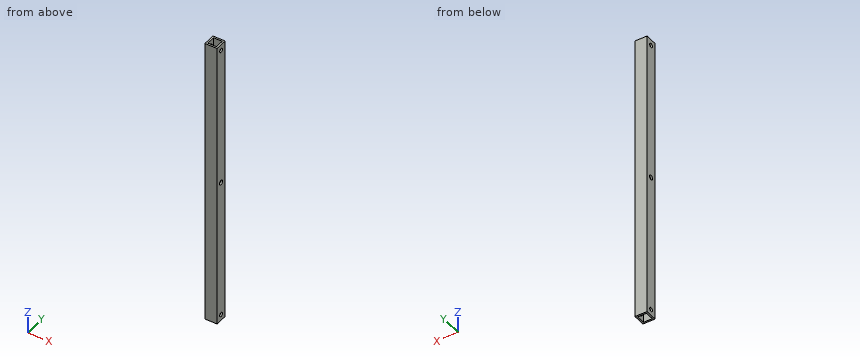
Autodesk Inventor part; units mm, degrees
ref_plane "YZ Plane" through (0, 0, 0) normal (1, 0, 0) x (0, 1, 0)
ref_plane "XZ Plane" through (0, 0, 0) normal (0, 1, 0) x (-1, 0, 0)
ref_plane "XY Plane" through (0, 0, 0) normal (0, 0, 1) x (1, 0, 0)
sketch "Sketch1" plane through (0, 0, 0) normal (0, 0, 1) x (1, 0, 0)
  line L0 (-6.35, -6.35) -> (6.35, -6.35)
  line L1 (6.35, -6.35) -> (6.35, 6.35)
  line L2 (6.35, 6.35) -> (-6.35, 6.35)
  line L3 (-6.35, 6.35) -> (-6.35, -6.35)
  line L4 (-6.35, -6.35) -> (6.35, 6.35) construction
  line L5 (6.35, -6.35) -> (-6.35, 6.35) construction
  line L6 (-4.572, -4.572) -> (4.572, -4.572)
  line L7 (4.572, -4.572) -> (4.572, 4.572)
  line L8 (4.572, 4.572) -> (-4.572, 4.572)
  line L9 (-4.572, 4.572) -> (-4.572, -4.572)
  line L10 (-4.572, -4.572) -> (4.572, 4.572) construction
  line L11 (4.572, -4.572) -> (-4.572, 4.572) construction
  point P0 (0, 0)
  dimension "d0" = 12.7
  dimension "d1" = 12.7
  dimension "d5" = 1.778
extrude "Extrusion1" add sketch "Sketch1" along normal blind 304.8
sketch "Sketch3" plane through (6.35, 6.35, 304.8) normal (1, 0, 0) x (0, 0, -1)
  point P0 (304.8, -6.35)
  point P1 (152.4, -6.35)
hole "Hole1" at (6.35, 0, 152.4) direction (-1, 0, 0) diameter 4.7625 depth 25.4 tip angle 118
sketch "Sketch4" plane through (-6.35, -6.35, 0) normal (-1, 0, 0) x (0, 0, 1)
  line L0 (0, 12.7) -> (0, 0)
  line L1 (304.8, 12.7) -> (304.8, 0)
  circle A0 centre (298.45, 6.35) radius 2.1336
  circle A1 centre (6.35, 6.35) radius 2.1336
  point P0 (0, 6.35)
  dimension "d13" = 4.2672
  dimension "d14" = 6.35
  dimension "d15" = 4.2672
  dimension "d16" = 6.35
extrude "Extrusion2" cut sketch "Sketch4" against normal blind 12.7
properties part number "5x5mm Box Aluminum" material "Aluminum 6061"
Part model, mm, in its own coordinate system. Give positions to 0.01 mm unless a question says otherwise; leave off trailing zeros. Loops run counter-clockwise (first coordinate to the right, second up) from the corner with the lowest first, then second, coordinate; pieces in that order, holes last. Notation, with made-up numbers: (5, 26) -> (18, 26) arc R25 ccw to (18, 55) -> close; hole circle Ø2 at (89, 5). An arc over 180 degrees is marked (long way). Write each question's results on one line, items separated by ' | '. Start each with the question number.
Q1. Wall check: L1, parallel to Y at x = 0, z = 268; L2, parallel to Y at x = -5.85, z = 6.35. Give the ranges that are in metal, low to high.
Q2. Band-saw the part on B-B on y = 0. Count the separate pieces of the cut face and the enclosed holes in it, plus the area to 3 significant figures.
Q3. Band-saw the part on A-A on x = 2.5. List the corners of the cut face in (y, z), plus the area to 3 significant figures.
Q4. Band-saw the part on C-C on z = 158.5. List the corners of the cut face in (x, y), plus the area to 3 significant figures.
Results are:
1) L1: y = -6.35 to -4.57, 4.57 to 6.35 | L2: y = -6.35 to -2.13, 2.13 to 6.35
2) separate pieces: 8 | enclosed holes: 0 | area: 1,040 mm²
3) outline: (-6.35, 0) -> (-4.57, 0) -> (-4.57, 304.8) -> (-6.35, 304.8) -> close; (4.57, 0) -> (6.35, 0) -> (6.35, 304.8) -> (4.57, 304.8) -> close | area: 1,080 mm²
4) outline: (-6.35, -6.35) -> (6.35, -6.35) -> (6.35, 6.35) -> (-6.35, 6.35) -> close; hole (-4.57, -4.57) -> (4.57, -4.57) -> (4.57, 4.57) -> (-4.57, 4.57) -> close | area: 77.7 mm²
